Autodesk Inventor part; units mm, degrees
ref_plane "YZ Plane" through (0, 0, 0) normal (1, 0, 0) x (0, 1, 0)
ref_plane "XZ Plane" through (0, 0, 0) normal (0, 1, 0) x (-1, 0, 0)
ref_plane "XY Plane" through (0, 0, 0) normal (0, 0, 1) x (1, 0, 0)
sketch "Sketch1" plane through (0, 0, 0) normal (0, 0, 1) x (1, 0, 0)
  line L0 (0, 0) -> (-65, 0)
  line L1 (-65, 0) -> (-65, 3.52)
  line L2 (0, 0) -> (0, 8.315)
  line L3 (0, 0) -> (0, 11.17)
  line L4 (0, 0) -> (15, 0)
  line L5 (15, 0) -> (15, 9.965)
  line L6 (15, 9.965) -> (0, 8.315)
  line L7 (0, 0) -> (-16.11, 0)
  line L8 (-16.11, 0) -> (-16.11, 7.185)
  line L9 (-16.11, 0) -> (-16.11, 10.455)
  line L10 (-65, 0) -> (-65, 6.275)
  line L11 (-65, 0) -> (-80.45, 0)
  line L12 (-80.45, 0) -> (-80.45, 2.625)
  line L13 (-80.45, 0) -> (-80.45, 5.16)
  line L14 (-80.45, 0) -> (-96.59, 0)
  line L15 (-96.59, 0) -> (-96.59, 1.65)
  line L16 (-65, 6.275) -> (-80.45, 5.16)
  line L17 (-96.59, 1.65) -> (-80.45, 2.625)
  line L18 (-65, 3.52) -> (-16.11, 7.185)
  line L19 (0, 11.17) -> (-16.11, 10.455)
  line L20 (-65, 0) -> (-65, -3.52)
  line L21 (0, 0) -> (0, -8.315)
  line L22 (0, 0) -> (0, -11.17)
  line L23 (15, 0) -> (15, -9.965)
  line L24 (15, -9.965) -> (0, -8.315)
  line L25 (-16.11, 0) -> (-16.11, -7.185)
  line L26 (-16.11, 0) -> (-16.11, -10.455)
  line L27 (-65, 0) -> (-65, -6.275)
  line L28 (-80.45, 0) -> (-80.45, -2.625)
  line L29 (-80.45, 0) -> (-80.45, -5.16)
  line L30 (-96.59, 0) -> (-96.59, -1.65)
  line L31 (-65, -6.275) -> (-80.45, -5.16)
  line L32 (-96.59, -1.65) -> (-80.45, -2.625)
  line L33 (-65, -3.52) -> (-16.11, -7.185)
  line L34 (0, -11.17) -> (-16.11, -10.455)
  point P0 (-16.11, -7.185)
  dimension "d0" = 65
  dimension "d1" = 3.52
  dimension "d2" = 8.315
  dimension "d3" = 11.17
  dimension "d4" = 15
  dimension "d6" = 9.965
  dimension "d7" = 16.11
  dimension "d8" = 7.185
  dimension "d9" = 10.455
  dimension "d10" = 6.275
  dimension "d11" = 15.45
  dimension "d12" = 2.625
  dimension "d13" = 5.16
  dimension "d14" = 16.14
  dimension "d15" = 1.65
extrude "Extrusion1" add sketch "Sketch1" along normal blind 3
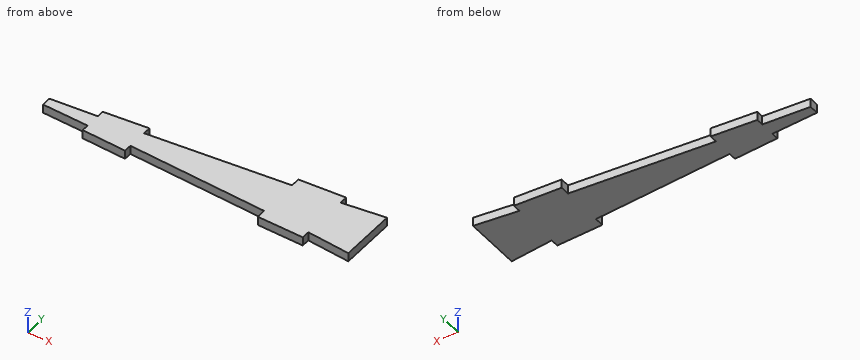
Could you check a few things on this model? Use its own coordinates, in mm. Give positions to 0.01 mm unless a question says otherwise; leave off trailing zeros. Loops run counter-clockwise (first coordinate to the right, second up) from the corner with the lowest first, then second, coordinate; pieces in that order, holes last. Notation, with made-up numbers: (78.25, 21) -> (97.25, 21) arc R14 cw to (97.25, 42) -> close; hole circle Ø10 at (-26, -4.75). An arc over 180 degrees is marked (long way). Put each result on its own line as item: value.
(1) Imagine slicing it at A-A on z = 1.35. Write out the boundary of the cut face in (x, y) (3 decimals), plus the area to 3 significant figures.
Computed:
outline: (-96.59, -1.65) -> (-80.45, -2.625) -> (-80.45, -5.16) -> (-65, -6.275) -> (-65, -3.52) -> (-16.11, -7.185) -> (-16.11, -10.455) -> (0, -11.17) -> (0, -8.315) -> (15, -9.965) -> (15, 9.965) -> (0, 8.315) -> (0, 11.17) -> (-16.11, 10.455) -> (-16.11, 7.185) -> (-65, 3.52) -> (-65, 6.275) -> (-80.45, 5.16) -> (-80.45, 2.625) -> (-96.59, 1.65) -> close
area: 1,390 mm^2
(2) Imagine slicing it at B-B on x = -84. Write out the boundary of the cut face in (y, z), plus the area to 3 significant figures.
Computed:
outline: (-2.41, 0) -> (2.41, 0) -> (2.41, 3) -> (-2.41, 3) -> close
area: 14.5 mm^2
(3) Imagine slicing it at C-C on x = 2. Write out the boundary of the cut face in (y, z) (3 decimals).
Computed:
outline: (-8.535, 0) -> (8.535, 0) -> (8.535, 3) -> (-8.535, 3) -> close
(4) Please list where these lines run through material, in increasing order: probe 1 along X at (y, z) = (-3, 2.2); probe 2 along Y at (x, z) = (-22, 0.6); probe 3 along Y at (x, z) = (-37, 0.4). Write a range as [from, to].
Computed:
probe 1: [-80.45, 15]
probe 2: [-6.74, 6.74]
probe 3: [-5.62, 5.62]
(5) I'm going to push flat-ended pins straight in: pin 1 Ø1.3 at (y, z) = (4.5, 2) entering from -X; pin 2 Ø0.9 at (y, z) = (8.5, 1) entering from -X; pin 3 Ø12 at (x, y) = (-82, 2) entering from -Z. Where does each tip first touch, or does it pass through?
Computed:
pin 1: x = -80.45
pin 2: x = -16.11
pin 3: z = 0
